Input: part model. Units: mm. Frame: model coordinates. Face numbers are marked on the shaded views. A direction names the side the tool comes from. Give positions to 0.01 mm unless a question says otherwise; leave off trailing zeros. Loops run counter-clockwise (first coordinate to the right, second up) from the corner with the lowest first, then second, coordinate; pieces in that order, holes last. Notation, with made-up numbers: M -28.75,27 L 9.25,27 A18 cw 9.25,51 Z; hole C -3.5,36 d2. An arc over 180 degrees is marked long. One line per item, written item: value. Start each with the question number.
(1) Ray query, line 1 along Y through (x, z) = (5, 74.5); line 2 along X through (y, z) = (115, 66.1); line 3 along X through (y, z) = (65, 68.45). Return the intervals inside material, ascending. Write a range as from..to.
(2) Pull-direction query (Y, two-part tool) for the marked faces 1, 2 and 3; classes: released by +Y, released by -Y, zero draft, split by the parting line, or undercut.
(3) Section A-A on y = 39. Output: boundary loops of the cut face in (x, z), plus the area to 3 significant figures.
(4) Section B-B on z = 72. Output: boundary loops of the cut face in (x, y), plus the area to 3 significant figures.
(5) Section C-C on x = 57.5. Output: boundary loops of the cut face in (y, z).
(6) Access query for the marked faces 4, 5, 6 and 7. Directions: +Z, -Z, +X, -X, +Y, -Y. A direction counts if a zero-diameter tool reaches every point of the face in a straight line with its end or side. Return the directions, or none.
(7) Pin query (flat end, axial travel): P1, Ø6.5, axis at x = 5.5, z = 76.5, coming from the +Y side; P2, Ø2.5, axis at x = 79, y = 115, coming from the +Z side; P3, Ø1.5, axis at x = 48.5, z = 69, coming from the -Y side; P4, Ø9, axis at y = 28, z = 75.5, coming from the -X side. Return the tip coordinate at first contact, or that it passes through.
(8) Section D-D on y = 23. Output: boundary loops of the cut face in (x, z).
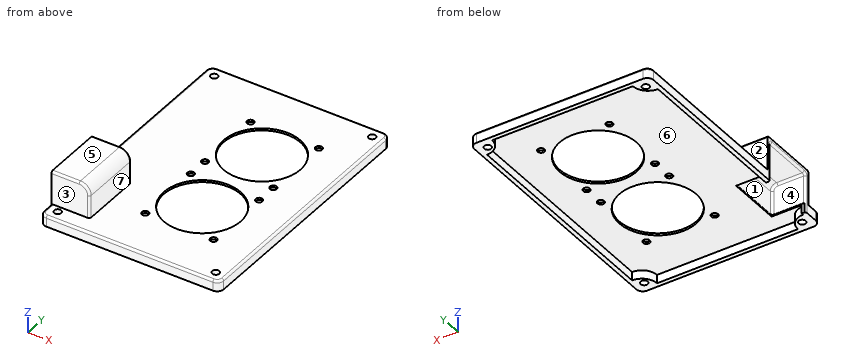
```python
from build123d import *

# Parameters (mm, degrees)
SKETCH009_R       = 1.65
PAD007_DEPTH      = 55
CYLINDER041_R     = 1.6
CYLINDER041_DEPTH = 10
CYLINDER042_R     = 18
CYLINDER042_DEPTH = 10
CYLINDER009_R     = 1.6
CYLINDER009_DEPTH = 10
CYLINDER010_R     = 18
CYLINDER010_DEPTH = 10
BOX016_W          = 18
BOX016_H          = 29
BOX016_DEPTH      = 16
FILLET020_R       = 5
THICKNESS_T       = -2.1
BOX015_W          = 18
BOX015_H          = 25
BOX015_DEPTH      = 18
PAD008_DEPTH      = 101
BOX010_W          = 84
BOX010_H          = 120
BOX010_DEPTH      = 5
FILLET012_R       = 3
FILLET034_R       = 1


with BuildPart() as pad007:
    # Sketch009 → Pad007 (new body)
    with BuildSketch(Plane.XY.offset(100)):
        with Locations((5, 115)):
            Circle(SKETCH009_R)
        with Locations((79, 115)):
            Circle(SKETCH009_R)
        with Locations((79, 5)):
            Circle(SKETCH009_R)
        with Locations((5, 5)):
            Circle(SKETCH009_R)
    extrude(amount=-PAD007_DEPTH)


with BuildPart() as cylinder041:
    # Cylinder041 → Cylinder041 (new body)
    with BuildSketch(Plane(origin=(-16, -16, 0), x_dir=(1, 0, 0), z_dir=(0, 0, 1))):
        Circle(CYLINDER041_R)
    extrude(amount=CYLINDER041_DEPTH)


with BuildPart() as part_mirroring003:
    # Part__Mirroring003: instance of Cylinder041
    add(cylinder041.part.mirror(Plane(origin=(0, 0, 0), x_dir=(1, 0, 0), z_dir=(0, 1, 0))))


with BuildPart() as part_mirroring005:
    # Part__Mirroring005: instance of Part__Mirroring003
    add(part_mirroring003.part.mirror(Plane(origin=(0, 0, 0), x_dir=(0, -1, 0), z_dir=(1, 0, 0))))


with BuildPart() as part_mirroring004:
    # Part__Mirroring004: instance of Cylinder041
    add(cylinder041.part.mirror(Plane(origin=(0, 0, 0), x_dir=(0, -1, 0), z_dir=(1, 0, 0))))


with BuildPart() as fusion040:
    # Cylinder042 → Cylinder042 (new body)
    with BuildSketch(Plane.XY):
        Circle(CYLINDER042_R)
    extrude(amount=CYLINDER042_DEPTH)

    # Fusion040: union Part__Mirroring003, Part__Mirroring005, Cylinder041, Part__Mirroring004
    add(part_mirroring003.part)
    add(part_mirroring005.part)
    add(cylinder041.part)
    add(part_mirroring004.part)


with BuildPart() as fusion040_1:
    # Fusion040 placement: moved
    add(fusion040.part.moved(Location((42, 40, 64))))


with BuildPart() as cylinder009:
    # Cylinder009 → Cylinder009 (new body)
    with BuildSketch(Plane(origin=(-16, -16, 0), x_dir=(1, 0, 0), z_dir=(0, 0, 1))):
        Circle(CYLINDER009_R)
    extrude(amount=CYLINDER009_DEPTH)


with BuildPart() as part_mirroring:
    # Part__Mirroring: instance of Cylinder009
    add(cylinder009.part.mirror(Plane(origin=(0, 0, 0), x_dir=(1, 0, 0), z_dir=(0, 1, 0))))


with BuildPart() as part_mirroring002:
    # Part__Mirroring002: instance of Part__Mirroring
    add(part_mirroring.part.mirror(Plane(origin=(0, 0, 0), x_dir=(0, -1, 0), z_dir=(1, 0, 0))))


with BuildPart() as part_mirroring001:
    # Part__Mirroring001: instance of Cylinder009
    add(cylinder009.part.mirror(Plane(origin=(0, 0, 0), x_dir=(0, -1, 0), z_dir=(1, 0, 0))))


with BuildPart() as fusion041:
    # Cylinder010 → Cylinder010 (new body)
    with BuildSketch(Plane.XY):
        Circle(CYLINDER010_R)
    extrude(amount=CYLINDER010_DEPTH)

    # Fusion009: union Part__Mirroring, Part__Mirroring002, Cylinder009, Part__Mirroring001
    add(part_mirroring.part)
    add(part_mirroring002.part)
    add(cylinder009.part)
    add(part_mirroring001.part)


with BuildPart() as fusion041_1:
    # Fusion009 placement: moved
    add(fusion041.part.moved(Location((42, 82, 64))))

    # Fusion041: union Fusion040
    add(fusion040_1.part)


with BuildPart() as fusion041_2:
    # Fusion041 placement: moved
    add(fusion041_1.part.moved(Location((8, -1, 0))))


with BuildPart() as thickness:
    # Box016 → Box016 (new body)
    with BuildSketch(Plane(origin=(0, 8, 68.5), x_dir=(1, 0, 0), z_dir=(0, 0, 1))):
        with Locations((9, 14.5)):
            Rectangle(BOX016_W, BOX016_H)
    extrude(amount=BOX016_DEPTH)

    # Fillet020
    fillet020_edges = [thickness.edges().sort_by_distance(p)[0] for p in [
        (18, 22.5, 84.5),
    ]]
    fillet(fillet020_edges, radius=FILLET020_R)

    # Thickness
    thickness_openings = [thickness.faces().sort_by_distance(p)[0] for p in [
        (0, 22.5, 76.5),
        (9, 22.5, 68.5),
    ]]
    offset(amount=THICKNESS_T, openings=thickness_openings)


with BuildPart() as cube015:
    # Box015 → Box015 (new body)
    with BuildSketch(Plane(origin=(-2, 10, 63), x_dir=(1, 0, 0), z_dir=(0, 0, 1))):
        with Locations((9, 12.5)):
            Rectangle(BOX015_W, BOX015_H)
    extrude(amount=BOX015_DEPTH)


with BuildPart() as pad008:
    # Sketch010 → Pad008 (new body)
    with BuildSketch(Plane.XY.offset(68)):
        with BuildLine():
            Line((82, 111), (82, 9))
            ThreePointArc((82, 9), (77.050253, 6.949747), (75, 2))
            Line((75, 2), (9, 2))
            ThreePointArc((9, 2), (6.949747, 6.949747), (2, 9))
            Line((2, 9), (2, 111))
            ThreePointArc((2, 111), (6.949747, 113.050253), (9, 118))
            Line((9, 118), (75, 118))
            ThreePointArc((75, 118), (77.050253, 113.050253), (82, 111))
        make_face()
    extrude(amount=-PAD008_DEPTH)


with BuildPart() as fillet034:
    # Box010 → Box010 (new body)
    with BuildSketch(Plane.XY.offset(64)):
        with Locations((42, 60)):
            Rectangle(BOX010_W, BOX010_H)
    extrude(amount=BOX010_DEPTH)

    # Fillet012
    fillet012_edges = [fillet034.edges().sort_by_distance(p)[0] for p in [
        (0, 0, 66.5),
        (0, 120, 66.5),
        (84, 0, 66.5),
        (84, 120, 66.5),
    ]]
    fillet(fillet012_edges, radius=FILLET012_R)

    # Cut014: cut Pad008
    add(pad008.part, mode=Mode.SUBTRACT)

    # Cut043: cut Cube015
    add(cube015.part, mode=Mode.SUBTRACT)

    # Fusion042: union Thickness
    add(thickness.part)

    # Cut044: cut Fusion041
    add(fusion041_2.part, mode=Mode.SUBTRACT)

    # Cut045: cut Pad007
    add(pad007.part, mode=Mode.SUBTRACT)

    # Fillet034
    fillet034_edges = [fillet034.edges().sort_by_distance(p)[0] for p in [
        (0, 34.9, 75.45),
        (0, 22.5, 82.4),
        (0, 10.1, 75.45),
        (15.05061, 10.1, 81.55061),
        (6.5, 34.9, 82.4),
        (0.87868, 119.12132, 69),
        (6.5, 8, 84.5),
        (6.5, 37, 84.5),
    ]]
    fillet(fillet034_edges, radius=FILLET034_R)


solid = fillet034.part
```
Output values:
1. line 1: y = 8..10.1, 34.9..37
1. line 2: x = 0..3.35, 6.65..8.32, 75.68..77.35, 80.65..84
1. line 3: x = 0.11..32.4, 35.6..41.75, 58.25..64.4, 67.6..83.89
2. face 1: undercut
2. face 2: released by +Y
2. face 3: released by -Y
3. outline: M 0,64 L 2,64 L 2,68 L 32,68 L 32,69 L 1,69 A1 ccw 0,68 Z; M 68,68 L 82,68 L 82,64 L 84,64 L 84,68 A1 ccw 83,69 L 68,69 Z
3. area: 63.6 mm²
4. outline: M 0,8 L 17,8 A1 ccw 18,9 L 18,36 A1 ccw 17,37 L 0,37 L 0,35.9 A1 ccw 1,34.9 L 14.9,34.9 A1 cw 15.9,33.9 L 15.9,11.1 A1 cw 14.9,10.1 L 1,10.1 A1 ccw 0,9.1 Z
4. area: 127 mm²
5. outline: M 0,64 L 2,64 L 2,68 L 22.64,68 L 22.64,69 L 1,69 A1 ccw 0,68 Z; M 55.36,68 L 64.64,68 L 64.64,69 L 55.36,69 Z; M 97.36,68 L 118,68 L 118,64 L 120,64 L 120,68 A1 ccw 119,69 L 97.36,69 Z
6. face 4: -Z, -X
6. face 5: +Z, +X, -X, +Y, -Y
6. face 6: -Z
6. face 7: +Z, +X, +Y, -Y
7. P1: stops at y = 37
7. P2: passes through
7. P3: stops at y = 0.03
7. P4: stops at x = 15.86
8. outline: M 0,83.4 A1 ccw 1,82.4 L 13,82.4 A2.9 cw 15.9,79.5 L 15.9,68.5 L 16,68.5 L 16,68 L 32.4,68 L 32.4,69 L 18,69 L 18,79.5 A5 ccw 13,84.5 L 0,84.5 Z; M 35.6,68 L 41.75,68 L 41.75,69 L 35.6,69 Z; M 58.25,68 L 64.4,68 L 64.4,69 L 58.25,69 Z; M 67.6,68 L 82,68 L 82,64 L 84,64 L 84,68 A1 ccw 83,69 L 67.6,69 Z
